```python
from build123d import *
from build123d.topology import SkipClean

# Parameters (mm, degrees)
SKETCH1_R               = 38.1
BOSS_EXTRUDE1_DEPTH     = 76.2
SHELL2_T                = 3.175
SKETCH2_W               = 3
SKETCH2_H               = 82.55
BOSS_EXTRUDE2_DEPTH     = 7
CUT_EXTRUDE1_DEPTH      = 99.527366122
CUT_EXTRUDE1_DEPTH_BACK = 99.527366122
SKETCH3_R               = 61.906276858
SKETCH3_R_2             = 41.275
SCALE1_SCALE            = 0.615384615


with BuildPart() as part:
    # Sketch1 → Boss-Extrude1 (new body)
    with BuildSketch(Plane(origin=(0, 0, 0), x_dir=(1, 0, 0), z_dir=(0, 1, 0))):
        with Locations(Location((0, 0, 0), (0, 0, 90))):
            Circle(SKETCH1_R)
    extrude(amount=BOSS_EXTRUDE1_DEPTH)

    # Shell2
    shell2_openings = [part.faces().sort_by_distance(p)[0] for p in [
        (0, 76.2, 0),
    ]]
    offset(amount=SHELL2_T, openings=shell2_openings, kind=Kind.INTERSECTION)

    # Sketch2 → Boss-Extrude2 (add)
    with BuildSketch(Plane(origin=(0, -3.175, 0), x_dir=(-1, 0, 0), z_dir=(0, -1, 0))):
        Rectangle(SKETCH2_W, SKETCH2_H)
        Polygon((-23.047310797, -34.273854321), (25.47436178, 32.510498564), (23.047310797, 34.273854321), (-25.47436178, -32.510498564), align=None)
        Polygon((-38.791332219, -14.181261217), (39.718383202, 11.328091668), (38.791332219, 14.181261217), (-39.718383202, -11.328091668), align=None)
        Polygon((-39.718383202, 11.328091668), (38.791332219, -14.181261217), (39.718383202, -11.328091668), (-38.791332219, 14.181261217), align=None)
        Polygon((-25.47436178, 32.510498564), (23.047310797, -34.273854321), (25.47436178, -32.510498564), (-23.047310797, 34.273854321), align=None)
    extrude(amount=BOSS_EXTRUDE2_DEPTH)

    # Sketch3 → Cut-Extrude1 (cut, two sides: drawn at the far end of the back side and taken through both)
    with SkipClean():  # the faces are left unmerged after this step: merging them gives an invalid solid
        with BuildSketch(Plane.XZ.offset(3.175).offset(-CUT_EXTRUDE1_DEPTH_BACK)):
            Circle(SKETCH3_R)
            with Locations(Location((0, 0, 0), (0, 0, 272.082679548))):
                Circle(SKETCH3_R_2, mode=Mode.SUBTRACT)
        extrude(amount=CUT_EXTRUDE1_DEPTH + CUT_EXTRUDE1_DEPTH_BACK, mode=Mode.SUBTRACT)


with BuildPart() as part_1:
    # Scale1: scaled about (0, 25.92844449, 0)
    add(part.part.scale(SCALE1_SCALE).moved(Location((0, 9.97247865, 0))))


solid = part_1.part
```
The model under review builds one solid part; all positions refer to its coordinate system, in mm. A direction names the side the tool comes from. Give positions to 0.01 mm unless a question says otherwise; leave off trailing zeros. Write each loop counter-clockwise with the first axis right and the second up, starting at its lowest first coordinate (ties: lowest second). Pieces come first, ordered by that corner, then holes. Notation, with made-up numbers: (81, 11.5) - (119, 11.5) arc R19 ccw to (119, 47.5) - close; hole circle Ø3 at (52, -40). An arc over 180 degrees is marked (long way). Answer in a Markdown table with one row per item. Add a question column.
1. Insertion check: P1, Ø4, axis at x = -8, y = 17, coming from the +Z side; P2, Ø4, axis at x = -10.5, z = 19.5, coming from the -Y side; P3, Ø1.3, axis at y = 5, z = 17.5, coming from the +X side. Each pin has a flat end and moves straight along its axis. Give the tip position at first contact, or say it passes through.
2. We need section D-D on z = 9.5. Write out the cut boundary in (x, y).
3. We need section B-B on x = 8. Write out the cut boundary in (y, z).
4. We need section A-A on y = 20. Write out the cut boundary in (x, z), then the cut area to 3 significant figures.
5. Tool access review of faces 1 (the flat face through (-17, 8.019, 0)), 2 (the flat face through (7.455, 5.895, -11.832)), 3 (the flat face through (-9.134, 5.895, 11.002)), 4 (the flat face through (-0.923, 6, 14)), 5 (the flat face through (17, 8.019, 0)): name each direction out of +Z, -Z, +X, -X, +Y, -Y from which nothing blocks a thin tool from reaching the whole face with its end or side.
6. We need section C-C on y = 9. Write out the cut boundary in (x, z), then the cut area to 3 significant figures.
7. Wall thickness on line 1 along X through (y, z) = (32, 0); line 2 along Z through (x, y) = (-0.5, 15.5); line 3 along Y through (x, z) = (-19.5, 12.5): over which ranges is each line inside the solid? List them lowest first. Write a range as [from, to].
Ans:
| question | item | result |
|---|---|---|
| 1 | P1 | stops at z = 24.68 |
| 1 | P2 | stops at y = 8.02 |
| 1 | P3 | stops at x = 14.33 |
| 2 | outline | (-23.56, 8.02) - (-8.04, 8.02) - (-8.04, 3.71) - (-5.76, 3.71) - (-5.76, 8.02) - (-0.92, 8.02) - (-0.92, 3.71) - (0.92, 3.71) - (0.92, 8.02) - (5.76, 8.02) - (5.76, 3.71) - (8.04, 3.71) - (8.04, 8.02) - (23.56, 8.02) - (23.56, 56.86) - (21.44, 56.86) - (21.44, 9.97) - (-21.44, 9.97) - (-21.44, 56.86) - (-23.56, 56.86) - close |
| 3 | outline | (3.71, -12.58) - (8.02, -12.58) - (8.02, -24.11) - (56.86, -24.11) - (56.86, -22.04) - (9.97, -22.04) - (9.97, 22.04) - (56.86, 22.04) - (56.86, 24.11) - (8.02, 24.11) - (8.02, 12.58) - (3.71, 12.58) - (3.71, 9.44) - (8.02, 9.44) - (8.02, 3.57) - (3.71, 3.57) - (3.71, 1.63) - (8.02, 1.63) - (8.02, -1.63) - (3.71, -1.63) - (3.71, -3.57) - (8.02, -3.57) - (8.02, -9.44) - (3.71, -9.44) - close |
| 4 | outline | circle Ø50.8 at (0, 0); hole circle Ø46.89 at (0, 0) |
| 4 | area | 300 mm^2 |
| 5 | face 1 | -X, -Y |
| 5 | face 2 | -Z, -Y |
| 5 | face 3 | -Y |
| 5 | face 4 | +Z, -Y |
| 5 | face 5 | +X, -Y |
| 6 | outline | circle Ø50.8 at (0, 0) |
| 6 | area | 2,030 mm^2 |
| 7 | line 1 | x = [-25.4, -23.45], [23.45, 25.4] |
| 7 | line 2 | z = [-25.4, -23.44], [23.44, 25.4] |
| 7 | line 3 | y = [8.02, 9.97] |
